Verification items for the finished model (mm, model axes). A direction names the side the tool comes from. Coordinates: 2 decimals unless noted, no trailing zeros. Loops run counter-clockwise (first coordinate to the right, second up) from the corner with the lowest first, then second, coordinate; pieces in that order, holes last. Notation, with made-up numbers: (20, 28) - (43, 28) arc R30 ccw to (43, 64) - close; hole circle Ø9 at (-5.5, 2.5). An arc over 180 degrees is marked (long way). Answer as CSV lines item,"result". Start each with the question number.
1. Material ranges on line 1 (X direction, y = 6.25, z = -6.5); line 2 (X direction, y = 19.25, z = -3); line 3 (Z direction, x = -5.25, y = 8), recorded low to high. Write a range as [from, to].
2. Cross-section at A-A (y = 16.75). Enter the section's corners in (x, z), plus the area to 3 significant figures.
3. Cross-section at B-B (x = 0). Enter the section's corners in (y, z), plus the area to 4 significant figures.
4. Cross-section at C-C (y = 8). Enter the section's corners in (x, z), plus the area to 3 significant figures.
5. Set-up check for faces 5 (the cylindrical face through (3.434, 19.574, 1.081)), 6 (the flat face through (6.521, 6.257, -0.492)), 7 (the flat face through (-6, 0, 0)), 8 (the flat face through (-7, 8, 2.8)), 9 (the flat face through (0, 18, -7)): record each of +Z, -Z, +X, -X, +Y, -Y from which the full face is reachable in a straight line by a thin tool's end or side.
6. Release check for a two-part mould opening along Z. For faces 1 (the flat face through (7.49, 12.68, -9.36)), 2 (the flat face through (8, 12, 0)), 3 (the flat face through (-7, 10.85, 0)), 4 (the flat face through (0, 21, 9.85)) record: pulls with the +Z half, pulls with the -Z half, needs draft (parallel to the pull), parting line crosses it, or undercut.
7. Gauge pin test, flat ends, axial feed: P1, Ø1.9, axis at x = 0, z = 0, coming from the -Y side; P2, Ø4.5, axis at y = 8, z = 0.5, coming from the -X side; P3, Ø3, axis at x = 1, z = 5, coming from the -Y side; P4, Ø1.5, axis at x = 4, z = 2.5, coming from the -Y side. Record the tip position at first contact, or that the pin passes through.
8. Cross-section at D-D (z = -8). Enter the section's corners in (x, y), plus the area to 3 significant figures.
Autodesk Inventor part; units mm, degrees
ref_plane "YZ Plane" through (0, 0, 0) normal (1, 0, 0) x (0, 1, 0)
ref_plane "XZ Plane" through (0, 0, 0) normal (0, 1, 0) x (-1, 0, 0)
ref_plane "XY Plane" through (0, 0, 0) normal (0, 0, 1) x (1, 0, 0)
sketch "Sketch3" plane through (0, 0, 0) normal (0, 1, 0) x (-1, 0, 0)
  line L0 (-8, 9.85) -> (8, 9.85)
  line L1 (8, 9.85) -> (8, -9.85)
  line L2 (8, -9.85) -> (-8, -9.85)
  line L3 (-8, -9.85) -> (-8, 9.85)
  line L4 (-8, 9.85) -> (8, -9.85) construction
  line L5 (8, 9.85) -> (-8, -9.85) construction
  line L6 (5, -9.85) -> (5, 9.85)
  line L7 (-5, 9.85) -> (-5, -9.85)
  line L8 (-5, -6.1562) -> (5, -6.1562) construction
  point P0 (0, 0)
  dimension "d12" = 19.7
  dimension "d36" = 10
  dimension "d52" = 16
extrude "Extrusion3" add sketch "Sketch3" along normal blind 25
sketch "Sketch4" plane through (8, 0, 9.85) normal (1, 0, 0) x (0, 0, -1)
  line L0 (9.85, 0) -> (9.85, 8) construction
  circle A0 centre (9.85, 8) radius 1.7
  line L1 (0, 0) -> (19.7, 0)
  line L2 (9.85, 5.9) -> (10.848, 6.6238)
  line L3 (8.852, 6.6238) -> (9.85, 5.9)
  dimension "d15" = 3.4
  dimension "d16" = 8
  dimension "d53" = 2.1
extrude "Extrusion4" cut sketch "Sketch3" along normal blind 18 contours L0 L6 L2 L7
extrude "Extrusion5" cut sketch "Sketch4" against normal through all
sketch "Sketch7" plane through (0, 25, 0) normal (0, 1, 0) x (1, 0, 0)
  circle A0 centre (0, 0) radius 1.6
  circle A1 centre (0, 0) radius 3.6
  line L0 (-5, 10) -> (5, -10) construction
  line L1 (8, 9.85) -> (-8, 9.85)
  line L2 (-8, 9.85) -> (-8, -9.85)
  line L3 (-8, -9.85) -> (8, -9.85)
  line L4 (8, -9.85) -> (8, 9.85)
  line L5 (-8, 9.85) -> (8, -9.85) construction
  line L6 (8, 9.85) -> (-8, -9.85) construction
  dimension "d30" = 3.2
  dimension "d47" = 7.2
extrude "Extrusion8" cut sketch "Sketch7" along normal through all both and the other way through all contours A0
extrude "Extrusion9" cut sketch "Sketch7" along normal blind 3 from surface at -7 contours A1
chamfer "Chamfer2" distance 2 angle 45 2 edges at (5, 18, 0) (-5, 18, 0)
chamfer "Chamfer3" distance 1 angle 45 4 edges at (-8, 12.5, 9.85) (-8, 12.5, -9.85) (8, 12.5, -9.85) (8, 12.5, 9.85)
sketch "Sketch9" plane through (-8, 0, -8.85) normal (-1, 0, 0) x (0, 0, 1)
  arc A0 (9.848, 6.6238) -> (7.852, 6.6238) centre (8.85, 8) ccw
  line L0 (6.05, 5.15) -> (11.65, 5.15)
  line L1 (11.65, 5.15) -> (11.65, 10.85)
  line L2 (11.65, 10.85) -> (6.05, 10.85)
  line L3 (6.05, 10.85) -> (6.05, 5.15)
  line L4 (6.05, 5.15) -> (11.65, 10.85) construction
  line L5 (11.65, 5.15) -> (6.05, 10.85) construction
  point P0 (8.85, 0)
  dimension "d57" = 5.6
  dimension "d58" = 5.7
extrude "Extrusion10" cut sketch "Sketch9" against normal blind 2.4
properties part number "Idlert Tensioner_3DPrint"
Values follow:
1,line 1,"x = [-8, -5], [5, 8]"
1,line 2,"x = [-8, -1.99], [1.99, 8]"
1,line 3,"z = [-9.85, -1.7], [1.7, 9.85]"
2,outline,"(-8, -8.85) - (-7, -9.85) - (-4.25, -9.85) - (-4.25, 9.85) - (-7, 9.85) - (-8, 8.85) - close; (4.25, -9.85) - (7, -9.85) - (8, -8.85) - (8, 8.85) - (7, 9.85) - (4.25, 9.85) - close"
2,area,"146 mm²"
3,outline,"(18, -9.85) - (25, -9.85) - (25, -1.6) - (21, -1.6) - (21, -3.6) - (18, -3.6) - close; (18, 3.6) - (21, 3.6) - (21, 1.6) - (25, 1.6) - (25, 9.85) - (18, 9.85) - close"
3,area,"103.5 mm²"
4,outline,"(-8, -8.85) - (-7, -9.85) - (-5, -9.85) - (-5, -1.7) - (-5.6, -1.7) - (-5.6, -2.8) - (-8, -2.8) - close; (-8, 2.8) - (-5.6, 2.8) - (-5.6, 1.7) - (-5, 1.7) - (-5, 9.85) - (-7, 9.85) - (-8, 8.85) - close; (5, -9.85) - (7, -9.85) - (8, -8.85) - (8, -1.7) - (5, -1.7) - close; (5, 1.7) - (8, 1.7) - (8, 8.85) - (7, 9.85) - (5, 9.85) - close"
4,area,"90.5 mm²"
5,face 5,"-Y"
5,face 6,"+X, -X"
5,face 7,"+Z, -Z, +X, -X, -Y"
5,face 8,"-X"
5,face 9,"+Z, -Z, -Y"
6,face 1,"pulls with the -Z half"
6,face 2,"needs draft"
6,face 3,"undercut"
6,face 4,"pulls with the +Z half"
7,P1,"passes through"
7,P2,"stops at x = -5.6"
7,P3,"stops at y = 18"
7,P4,"stops at y = 16.25"
8,outline,"(-8, 0) - (-5, 0) - (-5, 16) - (-3, 18) - (3, 18) - (5, 16) - (5, 0) - (8, 0) - (8, 25) - (-8, 25) - close"
8,area,"224 mm²"
